```python
from build123d import *

# Parameters (mm, degrees)
SKETCH_1_W          = 83
SKETCH_1_H          = 20
EXTRUDE_1_DEPTH     = 16
SKETCH_2_R          = 4
CUT_EXTRUDE_1_DEPTH = 3.5
SKETCH_3_R          = 1
CUT_EXTRUDE_2_DEPTH = 10
SKETCH_6_R          = 1
CUT_EXTRUDE_5_DEPTH = 8


with BuildPart() as part:
    # 스케치1 → 보스-돌출1 (new body)
    with BuildSketch(Plane(origin=(0, 0, 0), x_dir=(1, 0, 0), z_dir=(0, 1, 0))):
        Rectangle(SKETCH_1_W, SKETCH_1_H)
    extrude(amount=EXTRUDE_1_DEPTH)

    # 스케치2 → 컷-돌출1 (cut)
    with BuildSketch(Plane.XY.offset(10)):
        with Locations((-35.5, 10.5)):
            Circle(SKETCH_2_R)
        with Locations((35.5, 10.5)):
            Circle(SKETCH_2_R)
    extrude(amount=-CUT_EXTRUDE_1_DEPTH, mode=Mode.SUBTRACT)

    # 스케치3 → 컷-돌출2 (cut)
    with BuildSketch(Plane(origin=(0, 16, 0), x_dir=(1, 0, 0), z_dir=(0, 1, 0))):
        with Locations(Location((-25.5, -2, 0), (0, 0, 270))):
            Circle(SKETCH_3_R)
        with Locations(Location((25.5, -2, 0), (0, 0, 270))):
            Circle(SKETCH_3_R)
    extrude(amount=-CUT_EXTRUDE_2_DEPTH, mode=Mode.SUBTRACT)

    # 스케치6 → 컷-돌출5 (cut)
    with BuildSketch(Plane.XY.offset(6.5)):
        with Locations((-35.5, 10.5)):
            Circle(SKETCH_6_R)
        with Locations((35.5, 10.5)):
            Circle(SKETCH_6_R)
    extrude(amount=-CUT_EXTRUDE_5_DEPTH, mode=Mode.SUBTRACT)


solid = part.part
```
CAD build for the part. Positions are in the model's coordinates, mm. A direction names the side the tool comes from. Give positions to 0.01 mm unless a question says otherwise; leave off trailing zeros. Order: outer loops, then holes, each group sorted by start corner. A loop starts at its lowest first (then second) coordinate and runs counter-clockwise, first axis right, second up. Notation, with made-up numbers: M -23.75,-17 L 16.25,-17 A23 cw 16.25,6 Z; hole C 24.25,87 d6. An arc over 180 degrees is marked long. Put each result on its own line as item: value. Start each with the question number.
(1) Saw through at C-C, the plane x = -35.5. Write the cut outline in (y, z).
(2) Drill centre lines: line 1 along Y through (x, z) = (-35.5, 2.5); line 2 along Y through (x, z) = (35.5, 8.9); line 3 along X through (y, z) = (7.75, 7.75). Where is each one in solid material? Low to high.
(3) Which spindle directions (+Z, -Z, +X, -X, +Y, -Y) get a long thin tool onto all of the face, cutting with end or side? Do faces 4 (the flat face through (35, 11, -1.5)), 5 (the flat face through (-41.5, 8, 0)), 6 (the cylindrical face through (24.61, 11.07, 2.46)). Say none if no direction does.
(4) Flat gauge pins, fed straight in: pin 1 Ø0.6 at (x, y) = (36, 10.5) entering from +Z; pin 2 Ø6.5 at (x, y) = (-35.5, 10.5) entering from +Z; pin 3 Ø0.6 at (x, z) = (25.5, 2.5) entering from +Y. Where does each tip first touch, or does it go through?
(5) Saw through at A-A, the plane z = 2. Write the cut outline in (x, y), then the cut area to 3 significant figures.
(6) Saw through at B-B, the plane y = 10.5. Write the cut outline in (x, z), then the cut area to 3 significant figures.
(7) Saw through at D-D, the plane z = 8.25. Write the cut outline in (x, y).
(8) Mould opens along X. For faces 1 (the flat face through (41.5, 8, 0)), 2 (the cylindrical face through (32.55, 13.2, 8.27)), 3 (the flat face through (-1, 8, -10)) say: +X half, -X half, draft (parallel to the pull), parting line (faces both ways), or undercut.
Check result:
1. outline: M 0,-10 L 16,-10 L 16,10 L 14.5,10 L 14.5,6.5 L 11.5,6.5 L 11.5,-1.5 L 9.5,-1.5 L 9.5,6.5 L 6.5,6.5 L 6.5,10 L 0,10 Z
2. line 1: y = 0 to 9.5, 11.5 to 16
2. line 2: y = 0 to 6.5, 14.5 to 16
2. line 3: x = -41.5 to -38.4, -32.6 to 32.6, 38.4 to 41.5
3. face 4: +Z
3. face 5: +Z, -Z, -X, +Y, -Y
3. face 6: +Y
4. pin 1: stops at z = -1.5
4. pin 2: stops at z = 6.5
4. pin 3: stops at y = 6
5. outline: M -41.5,0 L 41.5,0 L 41.5,16 L 26.5,16 L 26.5,6 L 24.5,6 L 24.5,16 L -24.5,16 L -24.5,6 L -26.5,6 L -26.5,16 L -41.5,16 Z; hole C -35.5,10.5 d2; hole C 35.5,10.5 d2
5. area: 1,280 mm2
6. outline: M -41.5,-10 L 41.5,-10 L 41.5,10 L 39.5,10 L 39.5,6.5 L 36.5,6.5 L 36.5,-1.5 L 34.5,-1.5 L 34.5,6.5 L 31.5,6.5 L 31.5,10 L -31.5,10 L -31.5,6.5 L -34.5,6.5 L -34.5,-1.5 L -36.5,-1.5 L -36.5,6.5 L -39.5,6.5 L -39.5,10 L -41.5,10 Z; hole C -25.5,2 d2; hole C 25.5,2 d2
6. area: 1,570 mm2
7. outline: M -41.5,0 L 41.5,0 L 41.5,16 L -41.5,16 Z; hole C -35.5,10.5 d8; hole C 35.5,10.5 d8
8. face 1: +X half
8. face 2: undercut
8. face 3: draft
